Here's how the part is built. I have some questions about the finished solid (model axes, mm). A direction names the side the tool comes from. Round coordinates to 2 decimals unless told otherwise and drop trailing zeros. Write each loop counter-clockwise with the first axis right and the second up, starting at its lowest first coordinate (ties: lowest second). Pieces come first, ordered by that corner, then holes. Notation, with made-up numbers: (84, -4) -> (99, -4) arc R21 ccw to (99, 35) -> close; hole circle Ø11 at (86.5, 50.5). An arc over 180 degrees is marked (long way). Answer as CSV lines item,"result".
```python
from build123d import *

# Parameters (mm, degrees)
BOSS_EXTRUDE1_DEPTH             = 50
F_5_0MM_CLEARANCE_DOWEL_HOLE1_D = 5
CUT_EXTRUDE1_REACH              = 67.4
CUT_EXTRUDE1_END_RADIUS         = 31.75
SKETCH4_R                       = 5
CUT_EXTRUDE2_REACH              = 68.728
CUT_EXTRUDE2_END_RADIUS         = 31.75
CUT_EXTRUDE3_DEPTH              = 68.19468002
TAP_DRILL_FOR_M5X0_8_TAP1_D     = 4.2
TAP_DRILL_FOR_M5X0_8_TAP1_DEPTH = 8
TAP_DRILL_FOR_M5X0_8_TAP1_TIP   = 1.2618073


with BuildPart() as part:
    # Sketch1 → Boss-Extrude1 (new body)
    with BuildSketch(Plane.XY):
        with BuildLine():
            Line((-31.734248061, 1), (-17.721808598, 1))
            ThreePointArc((-17.721808598, 1), (0, 17.75), (17.721808598, 1))
            Line((17.721808598, 1), (31.734248061, 1))
            ThreePointArc((31.734248061, 1), (0, 31.75), (-31.734248061, 1))
        make_face()
    extrude(amount=BOSS_EXTRUDE1_DEPTH)

    # Ø5.0mm Clearance Dowel Hole1 (through all)
    with Locations(Plane(origin=(-24.72802833, 1, 40), x_dir=(0, 0, -1), z_dir=(0, -1, 0))):
        with Locations((0, 0), (30, 0), (0, 49.45605666), (30, 49.45605666)):
            Hole(F_5_0MM_CLEARANCE_DOWEL_HOLE1_D / 2)

    # Cut-Extrude1: up to this cylinder (the profile starts inside it)
    cut_extrude1_end = Plane(origin=(0, 0, 25), z_dir=(0, 0, -1)) * Cylinder(CUT_EXTRUDE1_END_RADIUS, 229.3, mode=Mode.PRIVATE)
    # Sketch4 → Cut-Extrude1 (cut, up to the surface)
    with BuildSketch(Plane(origin=(0, 4, 0), x_dir=(-1, 0, 0), z_dir=(0, -1, 0)), mode=Mode.PRIVATE) as cut_extrude1_sk1:
        with Locations(Location((24.72802833, -40, 0), (0, 0, 90))):
            Circle(SKETCH4_R)
    cut_extrude1_tool1 = extrude(cut_extrude1_sk1.sketch, amount=-CUT_EXTRUDE1_REACH, mode=Mode.PRIVATE) & cut_extrude1_end
    add(cut_extrude1_tool1.solids().sort_by_distance((-24.728028, 4, 40))[0], mode=Mode.SUBTRACT)
    # Sketch4 → Cut-Extrude1 (cut, up to the surface)
    with BuildSketch(Plane(origin=(0, 4, 0), x_dir=(-1, 0, 0), z_dir=(0, -1, 0)), mode=Mode.PRIVATE) as cut_extrude1_sk2:
        with Locations(Location((24.72802833, -10, 0), (0, 0, 90))):
            Circle(SKETCH4_R)
    cut_extrude1_tool2 = extrude(cut_extrude1_sk2.sketch, amount=-CUT_EXTRUDE1_REACH, mode=Mode.PRIVATE) & cut_extrude1_end
    add(cut_extrude1_tool2.solids().sort_by_distance((-24.728028, 4, 10))[0], mode=Mode.SUBTRACT)
    # Sketch4 → Cut-Extrude1 (cut, up to the surface)
    with BuildSketch(Plane(origin=(0, 4, 0), x_dir=(-1, 0, 0), z_dir=(0, -1, 0)), mode=Mode.PRIVATE) as cut_extrude1_sk3:
        with Locations(Location((-24.72802833, -10, 0), (0, 0, 90))):
            Circle(SKETCH4_R)
    cut_extrude1_tool3 = extrude(cut_extrude1_sk3.sketch, amount=-CUT_EXTRUDE1_REACH, mode=Mode.PRIVATE) & cut_extrude1_end
    add(cut_extrude1_tool3.solids().sort_by_distance((24.728028, 4, 10))[0], mode=Mode.SUBTRACT)
    # Sketch4 → Cut-Extrude1 (cut, up to the surface)
    with BuildSketch(Plane(origin=(0, 4, 0), x_dir=(-1, 0, 0), z_dir=(0, -1, 0)), mode=Mode.PRIVATE) as cut_extrude1_sk4:
        with Locations(Location((-24.72802833, -40, 0), (0, 0, 90))):
            Circle(SKETCH4_R)
    cut_extrude1_tool4 = extrude(cut_extrude1_sk4.sketch, amount=-CUT_EXTRUDE1_REACH, mode=Mode.PRIVATE) & cut_extrude1_end
    add(cut_extrude1_tool4.solids().sort_by_distance((24.728028, 4, 40))[0], mode=Mode.SUBTRACT)

    # Cut-Extrude2: up to this cylinder (the profile starts inside it)
    cut_extrude2_end = Plane(origin=(0, 0, 25), z_dir=(0, 0, -1)) * Cylinder(CUT_EXTRUDE2_END_RADIUS, 201.956, mode=Mode.PRIVATE)
    # Sketch5 → Cut-Extrude2 (cut, up to the surface)
    with BuildSketch(Plane(origin=(0, 1, 0), x_dir=(-1, 0, 0), z_dir=(0, -1, 0)), mode=Mode.PRIVATE) as cut_extrude2_sk1:
        with BuildLine():
            Line((-6, -35), (-6, -15))
            ThreePointArc((-6, -15), (0, -9), (6, -15))
            Line((6, -15), (6, -35))
            ThreePointArc((6, -35), (0, -41), (-6, -35))
        make_face()
    cut_extrude2_tool1 = extrude(cut_extrude2_sk1.sketch, amount=-CUT_EXTRUDE2_REACH, mode=Mode.PRIVATE) & cut_extrude2_end
    add(cut_extrude2_tool1.solids().sort_by_distance((0, 1, 25))[0], mode=Mode.SUBTRACT)

    # Sketch6 → Cut-Extrude3 (cut, through all)
    with BuildSketch(Plane.XY.offset(50)):
        with BuildLine():
            Line((18, 26.154588508), (-18, 26.154588508))
            ThreePointArc((-18, 26.154588508), (0, 31.75), (18, 26.154588508))
        make_face()
    extrude(amount=-CUT_EXTRUDE3_DEPTH, mode=Mode.SUBTRACT)

    # Tap Drill for M5x0.8 Tap1
    with Locations(Plane(origin=(-12.5, 26.154588508, 5), x_dir=(0, 0, 1), z_dir=(0, 1, 0))):
        with Locations((0, 0), (40, 0), (40, 25), (0, 25)):
            Hole(TAP_DRILL_FOR_M5X0_8_TAP1_D / 2, depth=TAP_DRILL_FOR_M5X0_8_TAP1_DEPTH)
            with Locations((0, 0, -(TAP_DRILL_FOR_M5X0_8_TAP1_DEPTH + TAP_DRILL_FOR_M5X0_8_TAP1_TIP / 2))):  # 118° drill point
                Cone(0, TAP_DRILL_FOR_M5X0_8_TAP1_D / 2, TAP_DRILL_FOR_M5X0_8_TAP1_TIP, mode=Mode.SUBTRACT)


solid = part.part
```
1. For pin 1 Ø6 at (x, z) = (2.5, 34) entering from -Y; pin 2 Ø5 at (x, z) = (23, 11) entering from +Y; pin 3 Ø5.5 at (x, z) = (12.5, 5) entering from +Y; pin 4 Ø3 at (x, z) = (23, 36) entering from +Y, each with a flat end and sliding along its axis, tell me the tip position at first contact or that it passes through.
Numbers:
pin 1,"passes through"
pin 2,"stops at y = 4"
pin 3,"stops at y = 26.15"
pin 4,"stops at y = 23.36"
2. If I drill on line 1 (Z direction, x = 12.5, y = 20.5); line 2 (Z direction, x = 13, y = 23.5); line 3 (X direction, y = 24.25, z = 5), over which ranges is the centre line in solid material (lowest first)?
Numbers:
line 1,"z = 0 to 2.9, 7.1 to 42.9, 47.1 to 50"
line 2,"z = 0 to 2.96, 7.04 to 42.96, 47.04 to 50"
line 3,"x = -20.49 to -14.6, -10.4 to 10.4, 14.6 to 20.49"
3. If we mould it in two halves opening along X, with no side actions, what happens to faces 4 (the face through (27.966, 15.032, 24.65)), 5 (the face through (19.847, 11.973, 11.084)), 6 (the face through (-25, 1, 25))? For each: released by +X, released by -X, zero draft, split by the parting line, or undercut.
Numbers:
face 4,"released by +X"
face 5,"undercut"
face 6,"zero draft"
4. Suppose I cut it at B-B on z = 20. Please give me the cut outline in (x, y), and give its area (3 significant figures).
Numbers:
outline,"(-31.73, 1) -> (-17.72, 1) arc R17.75 cw to (-6, 16.71) -> (-6, 26.15) -> (-18, 26.15) arc R31.75 ccw to start; (6, 16.71) arc R17.75 cw to (17.72, 1) -> (31.73, 1) arc R31.75 ccw to (18, 26.15) -> (6, 26.15) -> close"
area,"819 mm^2"
5. Suppose I cut it at D-D on x = 23. Please give me the cut outline in (y, z), and give its area (3 significant figures).
Numbers:
outline,"(1, 0) -> (21.89, 0) -> (21.89, 5.31) -> (4, 5.31) -> (4, 8.19) -> (1, 8.19) -> close; (1, 11.81) -> (4, 11.81) -> (4, 14.69) -> (21.89, 14.69) -> (21.89, 35.31) -> (4, 35.31) -> (4, 38.19) -> (1, 38.19) -> close; (1, 41.81) -> (4, 41.81) -> (4, 44.69) -> (21.89, 44.69) -> (21.89, 50) -> (1, 50) -> close"
area,"687 mm^2"
6. On a 3-axis mill with a long thin cutter (end or side, diameter ignored), from which of +Z, -Z, +X, -X, +Y, -Y can I reach the whole of each face in a straight line? I mean faces 1 (the face through (-6.215, 16.626, 24.65)), 2 (the face through (0, 21, 9)), 3 (the face through (-11.869, 22.099, 42.997)). Say none if no direction works.
Numbers:
face 1,"+Z, -Z, -Y"
face 2,"+Y, -Y"
face 3,"+Y"
7. Suppose I cut it at C-C on y = 6.5. Please give me the cut outline in (x, z).
Numbers:
outline,"(-31.08, 0) -> (-16.52, 0) -> (-16.52, 50) -> (-31.08, 50) -> close; (16.52, 0) -> (31.08, 0) -> (31.08, 50) -> (16.52, 50) -> close; hole circle Ø10 at (-24.73, 10); hole circle Ø10 at (-24.73, 40); hole circle Ø10 at (24.73, 10); hole circle Ø10 at (24.73, 40)"
8. Suppose I cut it at A-A on x = 0. Please give me the cut outline in (y, z).
Numbers:
outline,"(17.75, 0) -> (26.15, 0) -> (26.15, 9) -> (17.75, 9) -> close; (17.75, 41) -> (26.15, 41) -> (26.15, 50) -> (17.75, 50) -> close"
